Source: CAD feature listing. Evaluate the final solid. Frame: model axes, mm. A direction names the side the tool comes from. Give positions to 0.01 mm unless a question says otherwise; leave off trailing zeros. Order: outer loops, then holes, each group sorted by start corner. A loop starts at its lowest first (then second) coordinate and runs counter-clockwise, first axis right, second up. Notation, with made-up numbers: M 54.25,58 L 94.25,58 A20 ccw 94.25,83 Z; hole C 51,76.25 d7. An arc over 180 degrees is marked long. Use CSV: the item, a comma, the result in double quotes. Start each with the question number.
1. Section query C-C, the plane y = 14. Return the cut outline in (x, z).
2. Mould query, pull axis Z, two halves, no side actions, for faces 6 (the flat face through (19.5, 0, 16)), 7 (the flat face through (0, 17.5, 19)), 8 (the flat face through (0.29, 0.97, 54.59)), 9 (the flat face through (0.25, 16.65, 39.42)). Classes: released by +Z, released by -Z, zero draft, split by the parting line, or undercut.
3. Section query A-A, the plane x = 8.5. Return the cut outline in (y, z).
4. Section query D-D, the plane z = 47.5. Return the cut outline in (x, y).
5. Section query B-B, the plane z = 29.5. Return the cut outline in (x, y).
6. Reachability of faces 1 (the flat face through (-19.5, 3, 8)), 2 (the flat face through (0.21, 15.8, 41.66)), 3 (the flat face through (20.493, 8.699, 46.824)), 4 (the cylindrical face through (18.768, -0.583, 42.845)), 5 (the flat face through (-17.5, 0, 22)) from +Z, -Z, +X, -X, +Y, -Y: full face, straight path, thin tool, end or side. Return the list, or none.
7. Pin query (flat end, axial travel): P1, Ø6, axis at y = -14.5, z = 20, coming from the -X side; P2, Ø5, axis at x = 14.5, y = 4, coming from the +Z side; P3, Ø12, axis at x = 13, z = 48.5, coming from the +Y side. Return the tip coordinate at first contact, or that it passes through.
8. Line query: line 1 along Z through (x, y) = (18.1, 0); line 2 along Y through (x, z) = (3, 25.5); line 3 along Y through (x, z) = (2.5, 15). Output: solid intervals per line, ascending. Write a range as [from, to].
from build123d import *

# Parameters (mm, degrees)
F1_W      = 40
F1_H      = 40
F2_DEPTH  = 40
F5_DEPTH  = 40
F6_T      = -2.5
F4_W      = 22
F4_H      = 18
F7_DEPTH  = 0.5
F8_DEPTH  = 40
F9_W      = 35
F9_H      = 35
F10_DEPTH = 25
F11_W     = 22
F11_H     = 18
F12_DEPTH = 2.5
F13_W     = 5.9888265096
F13_H     = 10.6466971338
F14_DEPTH = 5
F15_DEPTH = 5
F17_DEPTH = 1
F18_W     = 9.2321382836
F18_H     = 9.3079488724
F18_W_2   = 12.2083812021
F18_H_2   = 12.2888814658
F18_W_3   = 13.6692405213
F18_H_3   = 15.1209759388
F19_DEPTH = 0.5
F20_DEPTH = 1
F21_W     = 9.1872019693
F21_H     = 7.9310182482
F21_W_2   = 24.7337101027
F21_H_2   = 9.711895138
F22_DEPTH = 0.5
F23_W     = 11.8269838858
F23_H     = 19.8296736926
F23_W_2   = 12.5252173748
F24_DEPTH = 0.5
F16_R     = 4.4787293466
F25_DEPTH = 2.5


with BuildPart() as f2:
    # F1 (on Top) → F2 (new body)
    with BuildSketch(Plane.XY):
        Rectangle(F1_W, F1_H)
    extrude(amount=F2_DEPTH)

    # F3 (on face) → F5 (join)
    with BuildSketch(Plane.YZ.offset(20)):
        Polygon((0, 55.334508419), (-20, 40), (20, 40), align=None)
    extrude(amount=-F5_DEPTH)

    # F6
    f6_openings = [f2.faces().sort_by_distance(p)[0] for p in [
        (0, 0, 0),
    ]]
    offset(amount=F6_T, openings=f6_openings)

    # F4 (on face) → F7 (cut)
    with BuildSketch(Plane.YZ.offset(20)):
        with Locations((0, 16)):
            Rectangle(F4_W, F4_H)
    extrude(amount=-F7_DEPTH, mode=Mode.SUBTRACT)

    # F3 (on face) → F8 (join)
    with BuildSketch(Plane.YZ.offset(20)):
        Polygon((20, 0), (-20, 0), (0, -8.4736328572), align=None)
    extrude(amount=-F8_DEPTH)

    # F9 (on Top) → F10 (cut)
    with BuildSketch(Plane.XY):
        Rectangle(F9_W, F9_H)
    extrude(amount=-F10_DEPTH, mode=Mode.SUBTRACT)

    # F11 (on face) → F12 (cut)
    with BuildSketch(Plane(origin=(0, 26.7190835157, 34.848307863), x_dir=(1, 0, 0), z_dir=(0, 0.6084609091, 0.7935838469))):
        with Locations((0.3634039909, -21.8104213327)):
            Rectangle(F11_W, F11_H)
    extrude(amount=-F12_DEPTH, mode=Mode.SUBTRACT)

    # F13 (on Right) → F14 (join)
    with BuildSketch(Plane.YZ):
        with Locations((-9.5960779581, 50.3422562033)):
            Rectangle(F13_W, F13_H)
    extrude(amount=F14_DEPTH)

    # F15 (cut): a face of the model
    f15_faces = [f2.faces().sort_by_distance(p)[0] for p in [
        (5, -7.5162341361, 45.7201312697),
    ]]
    extrude(f15_faces, amount=-F15_DEPTH, mode=Mode.SUBTRACT)

    # F16 (on face) → F17 (join)
    with BuildSketch(Plane.YZ.offset(20)):
        Polygon((0, 55.334508419), (-19.9640467717, 40.0275662541), (-17.6681634039, 40.0275662541), (0, 53.4335300326), (17.6441799849, 40.0275662541), (19.9640467717, 40.0275662541), align=None)
    extrude(amount=F17_DEPTH)

    # F18 (on face) → F19 (cut)
    with BuildSketch(Plane(origin=(-20, 0, 0), x_dir=(0, -1, 0), z_dir=(-1, 0, 0))):
        with Locations((-0.4024395021, 40.4120413586)):
            Rectangle(F18_W, F18_H)
        with Locations((8.3425419871, 25.8511127904)):
            Rectangle(F18_W_2, F18_H_2)
        with Locations((-3.3955307445, 7.5604879694)):
            Rectangle(F18_W_3, F18_H_3)
    extrude(amount=-F19_DEPTH, mode=Mode.SUBTRACT)

    # F18 (on face) → F20 (join)
    with BuildSketch(Plane(origin=(-20, 0, 0), x_dir=(0, -1, 0), z_dir=(-1, 0, 0))):
        Polygon((0, 55.334508419), (-20, 40), (-17.4968317151, 40), (0, 53.1819947064), (17.1925885671, 40), (20, 40), align=None)
    extrude(amount=F20_DEPTH)

    # F21 (on face) → F22 (cut)
    with BuildSketch(Plane(origin=(0, 20, 0), x_dir=(-1, 0, 0), z_dir=(0, 1, 0))):
        with Locations((-9.9281030707, 31.1322165653)):
            Rectangle(F21_W, F21_H)
        with Locations((2.3357556202, 15.6106483191)):
            Rectangle(F21_W_2, F21_H_2)
    extrude(amount=-F22_DEPTH, mode=Mode.SUBTRACT)

    # F23 (on face) → F24 (cut)
    with BuildSketch(Plane.XZ.offset(20)):
        with Locations((-8.3377951523, 20.714933984)):
            Rectangle(F23_W, F23_H)
        with Locations((9.1900789412, 20.714933984)):
            Rectangle(F23_W_2, F23_H)
    extrude(amount=-F24_DEPTH, mode=Mode.SUBTRACT)

    # F16 (on face) → F25 (cut)
    with BuildSketch(Plane.YZ.offset(20)):
        with Locations((0, 38.4044200182)):
            Circle(F16_R)
    extrude(amount=-F25_DEPTH, mode=Mode.SUBTRACT)


solid = f2.part
Result set:
1,outline,"M -21,42.63 L -20,42.63 L -20,-2.54 L -17.5,-2.54 L -17.5,41.45 L -10.64,41.45 L -10.64,44.6 L -21,44.6 Z; M 11.36,41.45 L 17.5,41.45 L 17.5,-2.54 L 20,-2.54 L 20,42.8 L 21,42.8 L 21,44.6 L 11.36,44.6 Z"
2,face 6,"undercut"
2,face 7,"zero draft"
2,face 8,"released by +Z"
2,face 9,"released by -Z"
3,outline,"M -20,0 L -17.5,-1.06 L -17.5,38.77 L 0,52.18 L 0.75,51.61 L 2.27,53.6 L 0,55.33 L -20,40 L -20,30.63 L -19.5,30.63 L -19.5,10.8 L -20,10.8 Z; M 15.03,40.66 L 17.5,38.77 L 17.5,-1.06 L 20,0 L 20,10.75 L 19.5,10.75 L 19.5,20.47 L 20,20.47 L 20,27.17 L 19.5,27.17 L 19.5,35.1 L 20,35.1 L 20,40 L 16.55,42.64 Z"
4,outline,"M -21,-10.22 L 0,-10.22 L 0,-12.59 L 5,-12.59 L 5,-10.22 L 21,-10.22 L 21,-7.82 L 20,-7.82 L 20,7.81 L 21,7.81 L 21,10.22 L 11.36,10.22 L 11.36,6.11 L 17.5,6.11 L 17.5,-6.11 L -17.5,-6.11 L -17.5,6.11 L -10.64,6.11 L -10.64,10.22 L -21,10.22 L -21,7.54 L -20,7.54 L -20,-7.41 L -21,-7.41 Z"
5,outline,"M -20,-20 L -14.25,-20 L -14.25,-19.5 L -2.42,-19.5 L -2.42,-20 L 2.93,-20 L 2.93,-19.5 L 15.45,-19.5 L 15.45,-20 L 20,-20 L 20,20 L 14.52,20 L 14.52,19.5 L 5.33,19.5 L 5.33,20 L -20,20 L -20,-2.24 L -19.5,-2.24 L -19.5,-14.45 L -20,-14.45 Z; hole M -17.5,-17.5 L 17.5,-17.5 L 17.5,17.5 L -17.5,17.5 Z"
6,face 1,"-X"
6,face 2,"+Z"
6,face 3,"-Z, +X"
6,face 4,"+X"
6,face 5,"-Z"
7,P1,"x = -20"
7,P2,"z = 54.18"
7,P3,"y = 16.74"
8,line 1,"[-8.47, 33.93], [42.88, 55.33]"
8,line 2,"[-19.5, -17.5], [17.5, 20]"
8,line 3,"[-20, -17.5], [17.5, 19.5]"
